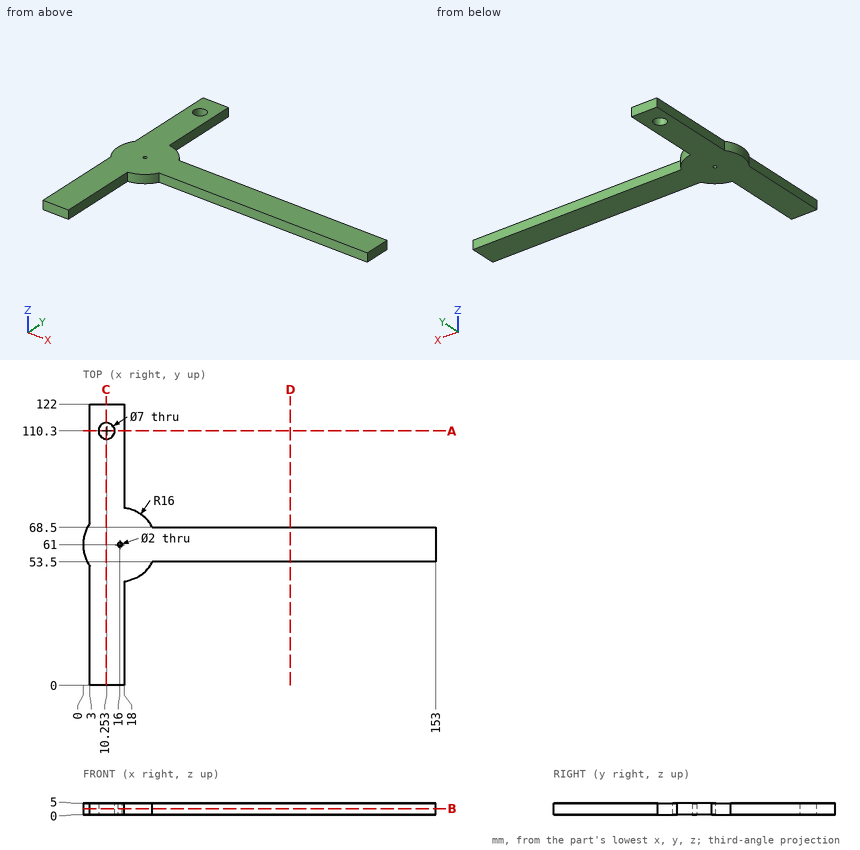
Print and shaded views of the part. All mm, measured from the part's lowest x, y and z. Round coordinates to 2 decimals unless told otherwise and drop trailing zeros. Write each loop counter-clockwise with the first axis right and the second up, starting at its lowest first coordinate (ties: lowest second). Pieces come first, ordered by that corner, then holes. Notation, with made-up numbers: (86, 53.25) -> (136, 53.25) arc R18 ccw to (136, 64.25) -> close; hole circle Ø2 at (53, -10). An arc over 180 degrees is marked (long way). Write item = value, one per line.
(1) Band-saw the part on C-C (x = 10). Give the cut face in (y, z).
Answer:
outline = (0, 0) -> (106.81, 0) -> (106.81, 5) -> (0, 5) -> close; (113.79, 0) -> (122, 0) -> (122, 5) -> (113.79, 5) -> close
(2) Band-saw the part on A-A (y = 110.3). Give the cut face in (x, z).
Answer:
outline = (3, 0) -> (6.75, 0) -> (6.75, 5) -> (3, 5) -> close; (13.75, 0) -> (18, 0) -> (18, 5) -> (13.75, 5) -> close
(3) Band-saw the part on B-B (z = 2.7). Give the cut face in (x, y) (1 decimal).
Answer:
outline = (3, 0) -> (18, 0) -> (18, 45.1) arc R16 ccw to (30.1, 53.5) -> (153, 53.5) -> (153, 68.5) -> (30.1, 68.5) arc R16 ccw to (18, 76.9) -> (18, 122) -> (3, 122) -> (3, 70.3) arc R16 ccw to (3, 51.7) -> close; hole circle Ø7 at (10.3, 110.3); hole circle Ø2 at (16, 61)
(4) Band-saw the part on D-D (x = 90). Give the cut face in (y, z), then the cut area to 3 significant figures.
Answer:
outline = (53.5, 0) -> (68.5, 0) -> (68.5, 5) -> (53.5, 5) -> close
area = 75.0 mm2
(5) Probe L1, parallel to Y at x = 73, z = 3.2; L2, parallel to X at y = 43.5, z = 2.5; L3, parallel to X at y = 63, z = 0.85 (1 decimal). List the from-to ranges inside material, lowest first.
Answer:
L1 = 53.5 to 68.5
L2 = 3 to 18
L3 = 0.1 to 153
(6) Flat gauge pins, fed straight in: pin 1 (1.5 mm diameter, centred on y = 15, z = 3.5, fed in from +X); pin 2 (2.5 mm diameter, centred on x = 103, z = 2.5, fed in from -Y); pin 3 (1.5 mm diameter, centred on x = 109.5, z = 2.5, fed in from +Y); pin 4 (5 mm diameter, centred on x = 18, y = 45.5, fed in from -Z). Where does each tip first touch, or does it go through?
Answer:
pin_1 = 18
pin_2 = 53.5
pin_3 = 68.5
pin_4 = 0
